Can you work these out from the model? Positions are in its coordinate system, mm. Face numbers are marked on the shaded views. A direction names the side the tool comes from. Give positions to 0.01 mm unless a question says otherwise; leave off trailing zeros. Order: outer loops, then holes, each group sorted by start corner. A loop starts at its lowest first (then second) coordinate and runs counter-clockwise, first axis right, second up.
Item 1: I want a section at B-B, the plane y = 281.5. Write out the boundary of the cut face in (x, z).
Item 2: I'm going to push flat-ended pins straight in: pin 1 Ø1.5 at (x, y) = (15.5, 268) entering from -Z; pin 2 Ø2.5 at (x, y) = (0, 269) entering from -Z; pin 3 Ø4.5 at (x, z) = (12, -21.5) entering from -Y. Where does each tip first touch, or does it pass through?
Item 3: I want a section at D-D, the plane y = 310. Write out the boundary of the cut face in (x, z), then the cut area to 4 significant figures.
Item 4: If I drill on line 1 along X through (y, z) = (274.5, -6); line 2 along X through (y, z) = (264.5, -6); line 3 along Y through (x, z) = (23, -7.5), over which ranges is the centre line in solid material (lowest first)?
Item 5: I want a section at C-C, the plane x = 27.5. Write out the boundary of the cut face in (y, z), then the cut area to 3 significant figures.
Item 6: Which directions (+Z, -Z, +X, -X, +Y, -Y) give clear straight access to the entire face, cutting with the end or side of a thin tool? Please do the marked faces 1, 2, 3 and 4.
Item 7: I want a section at A-A, the plane x = 8.25. Write out the boundary of the cut face in (y, z).
Item 8: If we mould it in two halves opening along Y, with no side actions, what happens to the marked faces 5, 6, 7 and 8? For each: +Y half, -Y half, draft (parallel to the pull), parting line (faces both ways), or undercut.
```python
from build123d import *

# Parameters (mm, degrees)
BOX005009018_W            = 20
BOX005009018_H            = 10
BOX005009018_DEPTH        = 26
BOX005009017_W            = 20
BOX005009017_H            = 33
BOX005009017_DEPTH        = 26
CYLINDER027_R             = 3
CYLINDER027_DEPTH         = 4
BOX005009016_W            = 16
BOX005009016_H            = 5.6
BOX005009016_DEPTH        = 3
CYLINDER026_R             = 1.7
CYLINDER026_DEPTH         = 30
FUSION024_PITCH_ANGLE     = 90
FUSION024_PLACEMENT_ANGLE = 90
FUSION023_PITCH_ANGLE     = 90
FUSION023_PLACEMENT_ANGLE = 90
CYLINDER025_R             = 1.7
CYLINDER025_DEPTH         = 20
BOX005009015_W            = 3.4
BOX005009015_H            = 26
BOX005009015_DEPTH        = 20
CYLINDER024_R             = 1.7
CYLINDER024_DEPTH         = 20
BOX005009009_W            = 10
BOX005009009_H            = 4.4
BOX005009009_DEPTH        = 70
CYLINDER015_R             = 2.2
CYLINDER015_DEPTH         = 70
CYLINDER014_R             = 2.2
CYLINDER014_DEPTH         = 70
FUSION009_PITCH_ANGLE     = 90
FUSION011_PITCH_ANGLE     = 90
CYLINDER022_R             = 3
CYLINDER022_DEPTH         = 6
CYLINDER022_ROLL_ANGLE    = 90
CHAMFER014_SIZE           = 2.9
CHAMFER012_SIZE           = 2.9
CHAMFER010_SIZE           = 2.9
CHAMFER008_SIZE           = 2.9
BOX005009011_W            = 41
BOX005009011_H            = 60
BOX005009011_DEPTH        = 29
BOX005009010_W            = 38.5
BOX005009010_H            = 64
BOX005009010_DEPTH        = 29
CHAMFER026_SIZE           = 3
FILLET003_R               = 7
FILLET004_R               = 7


with BuildPart() as cube005:
    # Box005009018 → Box005009018 (new body)
    with BuildSketch(Plane(origin=(-17, 313, -27), x_dir=(1, 0, 0), z_dir=(0, 0, 1))):
        with Locations((10, 5)):
            Rectangle(BOX005009018_W, BOX005009018_H)
    extrude(amount=BOX005009018_DEPTH)


with BuildPart() as fusion027:
    # Box005009017 → Box005009017 (new body)
    with BuildSketch(Plane(origin=(-17, 294, -38), x_dir=(1, 0, 0), z_dir=(0, 0, 1))):
        with Locations((10, 16.5)):
            Rectangle(BOX005009017_W, BOX005009017_H)
    extrude(amount=BOX005009017_DEPTH)

    # Fusion027: union Cube005
    add(cube005.part)


with BuildPart() as cylinder018:
    # Cylinder027 → Cylinder027 (new body)
    with BuildSketch(Plane.XY):
        Circle(CYLINDER027_R)
    extrude(amount=CYLINDER027_DEPTH)


with BuildPart() as cube003:
    # Box005009016 → Box005009016 (new body)
    with BuildSketch(Plane(origin=(-3.2, -2.8, 18), x_dir=(1, 0, 0), z_dir=(0, 0, 1))):
        with Locations((8, 2.8)):
            Rectangle(BOX005009016_W, BOX005009016_H)
    extrude(amount=BOX005009016_DEPTH)


with BuildPart() as cylinder017:
    # Cylinder026 → Cylinder026 (new body)
    with BuildSketch(Plane.XY.offset(1)):
        Circle(CYLINDER026_R)
    extrude(amount=CYLINDER026_DEPTH)


with BuildPart() as m3_cavity001:
    # Fusion024 base: copy of Cylinder017
    add(cylinder017.part)

    # Fusion024: union Cylinder018, Cube003
    add(cylinder018.part)
    add(cube003.part)


with BuildPart() as m3_cavity001_1:
    # Fusion024 pitch: moved
    add(m3_cavity001.part.rotate(Axis((0, 0, 0), (0, 1, 0)), FUSION024_PITCH_ANGLE))


with BuildPart() as m3_cavity001_2:
    # Fusion024 placement: moved
    add(m3_cavity001_1.part.moved(Location((15, 249, -6))).rotate(Axis((15, 249, -6), (0, 0, 1)), FUSION024_PLACEMENT_ANGLE))


with BuildPart() as m3_cavity:
    # Fusion023 base: copy of Cylinder017
    add(cylinder017.part)

    # Fusion023: union Cylinder018, Cube003
    add(cylinder018.part)
    add(cube003.part)


with BuildPart() as m3_cavity_1:
    # Fusion023 pitch: moved
    add(m3_cavity.part.rotate(Axis((0, 0, 0), (0, 1, 0)), FUSION023_PITCH_ANGLE))


with BuildPart() as m3_cavity_2:
    # Fusion023 placement: moved
    add(m3_cavity_1.part.moved(Location((0, 249, -6))).rotate(Axis((0, 249, -6), (0, 0, 1)), FUSION023_PLACEMENT_ANGLE))


with BuildPart() as cylinder016:
    # Cylinder025 → Cylinder025 (new body)
    with BuildSketch(Plane(origin=(8.25, 293, -17), x_dir=(1, 0, 0), z_dir=(0, 0, 1))):
        Circle(CYLINDER025_R)
    extrude(amount=CYLINDER025_DEPTH)


with BuildPart() as cube002:
    # Box005009015 → Box005009015 (new body)
    with BuildSketch(Plane(origin=(6.55, 267, -17), x_dir=(1, 0, 0), z_dir=(0, 0, 1))):
        with Locations((1.7, 13)):
            Rectangle(BOX005009015_W, BOX005009015_H)
    extrude(amount=BOX005009015_DEPTH)


with BuildPart() as slider_screw_slot:
    # Cylinder024 → Cylinder024 (new body)
    with BuildSketch(Plane(origin=(8.25, 267, -17), x_dir=(1, 0, 0), z_dir=(0, 0, 1))):
        Circle(CYLINDER024_R)
    extrude(amount=CYLINDER024_DEPTH)

    # Fusion022: union Cylinder016, Cube002
    add(cylinder016.part)
    add(cube002.part)


with BuildPart() as cube001:
    # Box005009009 → Box005009009 (new body)
    with BuildSketch(Plane(origin=(0, -2.2, 0), x_dir=(1, 0, 0), z_dir=(0, 0, 1))):
        with Locations((5, 2.2)):
            Rectangle(BOX005009009_W, BOX005009009_H)
    extrude(amount=BOX005009009_DEPTH)


with BuildPart() as cylinder014:
    # Cylinder015 → Cylinder015 (new body)
    with BuildSketch(Plane(origin=(10, 0, 0), x_dir=(1, 0, 0), z_dir=(0, 0, 1))):
        Circle(CYLINDER015_R)
    extrude(amount=CYLINDER015_DEPTH)


with BuildPart() as cylinder013:
    # Cylinder014 → Cylinder014 (new body)
    with BuildSketch(Plane.XY):
        Circle(CYLINDER014_R)
    extrude(amount=CYLINDER014_DEPTH)


with BuildPart() as m4_slot001:
    # Fusion009 base: copy of Cylinder013
    add(cylinder013.part)

    # Fusion009: union Cube001, Cylinder014
    add(cube001.part)
    add(cylinder014.part)


with BuildPart() as m4_slot001_1:
    # Fusion009 pitch: moved
    add(m4_slot001.part.rotate(Axis((0, 0, 0), (0, 1, 0)), FUSION009_PITCH_ANGLE))


with BuildPart() as m4_slot001_2:
    # Fusion009 placement: moved
    add(m4_slot001_1.part.moved(Location((-26, 305.5, -13))))


with BuildPart() as fusion019:
    # Fusion011 base: copy of Cylinder013
    add(cylinder013.part)

    # Fusion011: union Cube001, Cylinder014
    add(cube001.part)
    add(cylinder014.part)


with BuildPart() as fusion019_1:
    # Fusion011 pitch: moved
    add(fusion019.part.rotate(Axis((0, 0, 0), (0, 1, 0)), FUSION011_PITCH_ANGLE))


with BuildPart() as fusion019_2:
    # Fusion011 placement: moved
    add(fusion019_1.part.moved(Location((-26, 318, -6))))

    # Fusion019: union M4 slot001
    add(m4_slot001_2.part)


with BuildPart() as lug:
    # Cylinder022 → Cylinder022 (new body)
    with BuildSketch(Plane.XY):
        Circle(CYLINDER022_R)
    extrude(amount=CYLINDER022_DEPTH)


with BuildPart() as lug_1:
    # Cylinder022 roll: moved
    add(lug.part.rotate(Axis((0, 0, 0), (1, 0, 0)), CYLINDER022_ROLL_ANGLE))


with BuildPart() as lug_2:
    # Cylinder022 placement: moved
    add(lug_1.part.moved(Location((7.75, 328.8, -7))))


with BuildPart() as chamfer014:
    # Chamfer014 base: copy of lug
    add(lug_2.part)

    # Chamfer014
    chamfer014_edges = [chamfer014.edges().sort_by_distance(p)[0] for p in [
        (4.75, 328.8, -7),
    ]]
    chamfer(chamfer014_edges, length=CHAMFER014_SIZE)


with BuildPart() as chamfer014_1:
    # Chamfer014 placement: moved
    add(chamfer014.part.moved(Location((6, -1, 0))))


with BuildPart() as part_mirroring002:
    # Part__Mirroring002: instance of Chamfer014
    add(chamfer014_1.part.mirror(Plane(origin=(0, 200, 0), x_dir=(1, 0, 0), z_dir=(0, 1, 0))))


with BuildPart() as chamfer012:
    # Chamfer012 base: copy of lug
    add(lug_2.part)

    # Chamfer012
    chamfer012_edges = [chamfer012.edges().sort_by_distance(p)[0] for p in [
        (4.75, 328.8, -7),
    ]]
    chamfer(chamfer012_edges, length=CHAMFER012_SIZE)


with BuildPart() as chamfer012_1:
    # Chamfer012 placement: moved
    add(chamfer012.part.moved(Location((-6, -1, 0))))


with BuildPart() as fusion016:
    # Part__Mirroring: instance of Chamfer012
    add(chamfer012_1.part.mirror(Plane(origin=(0, 200, 0), x_dir=(1, 0, 0), z_dir=(0, 1, 0))))

    # Fusion016: union Part__Mirroring002
    add(part_mirroring002.part)


with BuildPart() as fusion016_1:
    # Fusion016 placement: moved
    add(fusion016.part.moved(Location((0, 186, 0))))


with BuildPart() as chamfer010:
    # Chamfer010 base: copy of lug
    add(lug_2.part)

    # Chamfer010
    chamfer010_edges = [chamfer010.edges().sort_by_distance(p)[0] for p in [
        (4.75, 328.8, -7),
    ]]
    chamfer(chamfer010_edges, length=CHAMFER010_SIZE)


with BuildPart() as chamfer010_1:
    # Chamfer010 placement: moved
    add(chamfer010.part.moved(Location((6, -1, 0))))


with BuildPart() as lugs:
    # Chamfer008 base: copy of lug
    add(lug_2.part)

    # Chamfer008
    chamfer008_edges = [lugs.edges().sort_by_distance(p)[0] for p in [
        (4.75, 328.8, -7),
    ]]
    chamfer(chamfer008_edges, length=CHAMFER008_SIZE)


with BuildPart() as lugs_1:
    # Chamfer008 placement: moved
    add(lugs.part.moved(Location((-6, -1, 0))))

    # Fusion014: union Chamfer010
    add(chamfer010_1.part)


with BuildPart() as slider002:
    # Box005009011 → Box005009011 (new body)
    with BuildSketch(Plane(origin=(-8, 238, -41.5), x_dir=(1, 0, 0), z_dir=(0, 0, 1))):
        with Locations((20.5, 30)):
            Rectangle(BOX005009011_W, BOX005009011_H)
    extrude(amount=BOX005009011_DEPTH)


with BuildPart() as slider_support:
    # Box005009010 → Box005009010 (new body)
    with BuildSketch(Plane(origin=(-7, 261, -31.5), x_dir=(1, 0, 0), z_dir=(0, 0, 1))):
        with Locations((19.25, 32)):
            Rectangle(BOX005009010_W, BOX005009010_H)
    extrude(amount=BOX005009010_DEPTH)

    # Cut015: cut slider002
    add(slider002.part, mode=Mode.SUBTRACT)

    # Fusion015: union lugs
    add(lugs_1.part)

    # Fusion018: union Fusion016
    add(fusion016_1.part)

    # Cut018: cut Fusion019
    add(fusion019_2.part, mode=Mode.SUBTRACT)

    # Cut022: cut slider-screw-slot
    add(slider_screw_slot.part, mode=Mode.SUBTRACT)

    # Chamfer026
    chamfer026_edges = [slider_support.edges().sort_by_distance(p)[0] for p in [
        (12.25, 298, -12.5),
    ]]
    chamfer(chamfer026_edges, length=CHAMFER026_SIZE)

    # Fillet003
    fillet003_edges = [slider_support.edges().sort_by_distance(p)[0] for p in [
        (12.25, 298, -31.5),
    ]]
    fillet(fillet003_edges, radius=FILLET003_R)

    # Fillet004
    fillet004_edges = [slider_support.edges().sort_by_distance(p)[0] for p in [
        (12.25, 325, -31.5),
    ]]
    fillet(fillet004_edges, radius=FILLET004_R)

    # Cut023: cut M3-cavity
    add(m3_cavity_2.part, mode=Mode.SUBTRACT)

    # Cut024: cut M3-cavity001
    add(m3_cavity001_2.part, mode=Mode.SUBTRACT)

    # Cut027: cut Fusion027
    add(fusion027.part, mode=Mode.SUBTRACT)


solid = slider_support.part
```
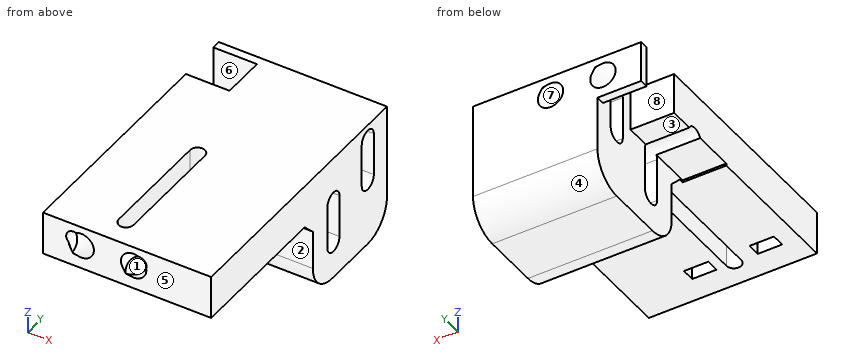
Results list:
1. outline: (-7, -12.5) - (6.55, -12.5) - (6.55, -2.5) - (-7, -2.5) - close; (9.95, -12.5) - (31.5, -12.5) - (31.5, -2.5) - (9.95, -2.5) - close
2. pin 1: stops at z = -2.8
2. pin 2: stops at z = -12.5
2. pin 3: stops at y = 298
3. outline: (-7, -12) - (3, -12) - (3, -31.5) - (31.5, -31.5) - (31.5, -2.5) - (-7, -2.5) - close
3. area: 921.5 mm2
4. line 1: x = -7 to -1.7, 1.7 to 6.55, 9.95 to 13.3, 16.7 to 31.5
4. line 2: x = -7 to -1.7, 1.7 to 13.3, 16.7 to 31.5
4. line 3: y = 261 to 315.8, 320.2 to 325
5. outline: (261, -12.5) - (295, -12.5) - (298, -15.5) - (298, -24.5) arc R7 ccw to (305, -31.5) - (318, -31.5) arc R7 ccw to (325, -24.5) - (325, -2.5) - (261, -2.5) - close; hole (303.3, -23) arc R2.2 ccw to (307.7, -23) - (307.7, -13) arc R2.2 ccw to (303.3, -13) - close; hole (315.8, -16) arc R2.2 ccw to (320.2, -16) - (320.2, -6) arc R2.2 ccw to (315.8, -6) - close
5. area: 1,020 mm2
6. face 1: -Y
6. face 2: -Z, +X, -X, -Y
6. face 3: -Z, -X, +Y
6. face 4: -Z, +X, -X, +Y
7. outline: (261, -12.5) - (265.3, -12.5) - (265.3, -2.5) - (261, -2.5) - close; (294.7, -12.5) - (295, -12.5) - (298, -15.5) - (298, -24.5) arc R7 ccw to (305, -31.5) - (318, -31.5) arc R7 ccw to (325, -24.5) - (325, -2.5) - (294.7, -2.5) - close; hole (303.3, -23) arc R2.2 ccw to (307.7, -23) - (307.7, -13) arc R2.2 ccw to (303.3, -13) - close; hole (315.8, -16) arc R2.2 ccw to (320.2, -16) - (320.2, -6) arc R2.2 ccw to (315.8, -6) - close
8. face 5: -Y half
8. face 6: undercut
8. face 7: +Y half
8. face 8: undercut
